Verification items for the finished model (mm, model axes). A direction names the side the tool comes from. Coordinates: 2 decimals unless noted, no trailing zeros. Write each loop counter-clockwise with the first axis right and the second up, starting at its lowest first coordinate (ties: lowest second). Pieces come first, ordered by that corner, then holes. Notation, with made-up numbers: (50.25, 49) -> (105.25, 49) arc R28 ccw to (105.25, 69) -> close; hole circle Ø4 at (0, -28.75). An arc over 180 degrees is marked (long way). Use CSV: the item, a comma, the result in double quotes.
```python
from build123d import *

# Parameters (mm, degrees)
F0_W     = 57
F0_H     = 92
F1_DEPTH = 90
F2_W     = 55
F2_H     = 90
F3_DEPTH = 89
F4_W     = 57
F4_H     = 91
F5_DEPTH = 45
F6_R     = 10
F7_DEPTH = 1
F8_R     = 2


with BuildPart() as f1:
    # F0 (on Top) → F1 (new body)
    with BuildSketch(Plane.XY):
        Rectangle(F0_W, F0_H)
    extrude(amount=F1_DEPTH)

    # F2 (on face) → F3 (cut)
    with BuildSketch(Plane.XY.offset(90)):
        Rectangle(F2_W, F2_H)
    extrude(amount=-F3_DEPTH, mode=Mode.SUBTRACT)

    # F4 (on face) → F5 (cut)
    with BuildSketch(Plane.XY.offset(90)):
        with Locations((0, 0.5)):
            Rectangle(F4_W, F4_H)
    extrude(amount=-F5_DEPTH, mode=Mode.SUBTRACT)

    # F6 (on face) → F7 (cut)
    with BuildSketch(Plane.XZ.offset(46)):
        with Locations((0, 44.787799)):
            Circle(F6_R)
    extrude(amount=-F7_DEPTH, mode=Mode.SUBTRACT)

    # F8
    f8_edges = [f1.edges().sort_by_distance(p)[0] for p in [
        (27.5, 0, 1),
        (0, 45, 1),
        (-27.5, 0, 1),
        (0, -45, 1),
    ]]
    fillet(f8_edges, radius=F8_R)


solid = f1.part
```
1) Mould release check, pull along X, two halves, no side actions. Record for faces 1 (the cylindrical face through (-1.302, -45.507, 54.703)), 2 (the flat face through (0, 1, 0)), 3 (the flat face through (-28.5, -1, 24)): released by +X, released by -X, zero draft, split by the parting line, or undercut.
Return value:
face 1,"undercut"
face 2,"zero draft"
face 3,"released by -X"
2) Set-up check for faces 4 (the flat face through (27.5, -1, 24)), 5 (the flat face through (-28, 1, 45)), 6 (the flat face through (0, 46, 22)): record each of +Z, -Z, +X, -X, +Y, -Y from which the full face is reachable in a straight line by a thin tool's end or side.
Return value:
face 4,"+Z"
face 5,"+Z, +X, -X, +Y"
face 6,"+Z, -Z, +X, -X, +Y"
3) Cross-section at D-D (x = -8). Record the boundary of the cut face in (y, z).
Return value:
outline,"(-46, 0) -> (46, 0) -> (46, 45) -> (45, 45) -> (45, 3) arc R2 cw to (43, 1) -> (-43, 1) arc R2 cw to (-45, 3) -> (-45, 38.79) -> (-46, 38.79) -> close; (-46, 50.79) -> (-45, 50.79) -> (-45, 90) -> (-46, 90) -> close"
4) Cross-section at C-C (y = -8.5). Record the boundary of the cut face in (x, z).
Return value:
outline,"(-28.5, 0) -> (28.5, 0) -> (28.5, 45) -> (27.5, 45) -> (27.5, 3) arc R2 cw to (25.5, 1) -> (-25.5, 1) arc R2 cw to (-27.5, 3) -> (-27.5, 45) -> (-28.5, 45) -> close"
5) Cross-section at B-B (z = 53). Record the boundary of the cut face in (x, y), plus the area to 3 significant figures.
Return value:
outline,"(-28.5, -46) -> (-5.71, -46) -> (-5.71, -45) -> (-28.5, -45) -> close; (5.71, -46) -> (28.5, -46) -> (28.5, -45) -> (5.71, -45) -> close"
area,"45.6 mm2"
6) Scan lines: L1, parallel to Z at x = 0, y = -45.3; L2, parallel to X at y = -8, z = 4.5; L3, parallel to Y at x = -1.5, z = 20.5. Record each from-to range of solid material in increasing order.
Return value:
L1,"0 to 34.79, 54.79 to 90"
L2,"-28.5 to -27.5, 27.5 to 28.5"
L3,"-46 to -45, 45 to 46"
7) Gauge pin test, flat ends, axial feed: pin 1 (6 mm diameter, centred on x = 3.5, y = -4.5, fed in from +Z); pin 2 (4 mm diameter, centred on x = 14, z = 81, fed in from +Y). Record the tip position at first contact, or that the pin passes through.
Return value:
pin 1,"z = 1"
pin 2,"y = -45"
8) Cross-section at A-A (x = 0). Record the boundary of the cut face in (y, z).
Return value:
outline,"(-46, 0) -> (46, 0) -> (46, 45) -> (45, 45) -> (45, 3) arc R2 cw to (43, 1) -> (-43, 1) arc R2 cw to (-45, 3) -> (-45, 34.79) -> (-46, 34.79) -> close; (-46, 54.79) -> (-45, 54.79) -> (-45, 90) -> (-46, 90) -> close"
